Geometry: final body of the model. Coordinates: model frame, mm. A direction names the side the tool comes from. Round coordinates to 2 decimals unless told otherwise and drop trailing zeros. Loops run counter-clockwise (first coordinate to the right, second up) from the corner with the lowest first, then second, coordinate; pieces in that order, holes last. Notation, with made-up numbers: M -21.5,73.5 L 23.5,73.5 A24 cw 23.5,91.5 Z; hole C 83.5,-22.75 d3. An arc over 180 degrees is marked long. Answer as a JSON object with one key per item and string values.
from build123d import *

# Parameters (mm, degrees)
F1_DEPTH = 3
F2_R     = 2.5
F3_DEPTH = 23


with BuildPart() as f1:
    # F0 (on Top) → F1 (new body)
    with BuildSketch(Plane.XY):
        with BuildLine():
            Line((8.3654914829, 7.7478343503), (8.3654914829, 25.7808157751))
            ThreePointArc((8.3654914829, 25.7808157751), (0.4767203504, 33.9966565171), (-7.631576467, 25.9973895632))
            Line((-7.631576467, 25.9973895632), (-8.6528857034, 7.4260866897))
            ThreePointArc((-8.6528857034, 7.4260866897), (-9.3855131516, 5.0826540918), (-11.1453419747, 3.3705145438))
            Line((-11.1453419747, 3.3705145438), (-26.7623619946, -5.6459761686))
            ThreePointArc((-26.7623619946, -5.6459761686), (-29.9331032244, -16.585772745), (-18.951386422, -19.6081302933))
            Line((-18.951386422, -19.6081302933), (-2.3575117339, -11.2069586004))
            ThreePointArc((-2.3575117339, -11.2069586004), (0.038274152, -10.6697162831), (2.400944907, -11.3377029763))
            Line((2.400944907, -11.3377029763), (18.0179649268, -20.3541936886))
            ThreePointArc((18.0179649268, -20.3541936886), (29.0774772891, -17.6302378543), (26.2040573041, -6.6086133521))
            Line((26.2040573041, -6.6086133521), (10.6314918524, 3.5615178285))
            ThreePointArc((10.6314918524, 3.5615178285), (8.9683334147, 5.3677081091), (8.3654914829, 7.7478343503))
        make_face()
        with BuildLine():
            ThreePointArc((-20.451386422, -12.679927063), (-25.3707248656, -13.3098488797), (-20.7688276181, -11.4607318089))
            ThreePointArc((-20.7688276181, -11.4607318089), (-20.5320479783, -12.0500052463), (-20.451386422, -12.679927063))
        make_face(mode=Mode.SUBTRACT)
        with BuildLine():
            ThreePointArc((24.7040573041, -13.5368165824), (21.5399163779, -15.9469860432), (20.0569238399, -12.25626284))
            ThreePointArc((20.0569238399, -12.25626284), (22.8681982302, -11.1266471215), (24.7040573041, -13.5368165824))
        make_face(mode=Mode.SUBTRACT)
        with BuildLine():
            ThreePointArc((-7.9164689421, -4.2812988086), (-7.6979940139, 4.6627125327), (0.127531223, 8.9990963873))
            ThreePointArc((0.127531223, 8.9990963873), (6.4088915191, 6.3187110629), (9, 0))
            ThreePointArc((9, 0), (8.6421794957, -2.5125153857), (7.5971703192, -4.8252464332))
            ThreePointArc((7.5971703192, -4.8252464332), (-0.315369081, -8.9944728774), (-7.9164689421, -4.2812988086))
        make_face(mode=Mode.SUBTRACT)
        with BuildLine():
            ThreePointArc((2.868423533, 25.9973895632), (2.1236210505, 24.217141919), (0.3329981933, 23.4976405667))
            ThreePointArc((0.3329981933, 23.4976405667), (-1.3867739845, 27.7776372074), (2.868423533, 25.9973895632))
        make_face(mode=Mode.SUBTRACT)
        with BuildLine():
            Line((7.5971703192, -4.8252464332), (2.0066709741, -1.4910639161))
            ThreePointArc((2.0066709741, -1.4910639161), (-0.2232494881, -2.4900119811), (-2.239906233, -1.1103243073))
            Line((-2.239906233, -1.1103243073), (-7.9164689421, -4.2812988086))
            ThreePointArc((-7.9164689421, -4.2812988086), (-0.315369081, -8.9944728774), (7.5971703192, -4.8252464332))
        make_face()
        with BuildLine():
            ThreePointArc((-2.239906233, -1.1103243073), (-2.1149683962, 1.333007383), (0.0354253397, 2.4997489965))
            Line((0.0354253397, 2.4997489965), (0.127531223, 8.9990963873))
            ThreePointArc((0.127531223, 8.9990963873), (-7.6979940139, 4.6627125327), (-7.9164689421, -4.2812988086))
            Line((-7.9164689421, -4.2812988086), (-2.239906233, -1.1103243073))
        make_face()
        with BuildLine():
            ThreePointArc((0.0354253397, 2.4997489965), (1.7802476442, 1.7551975175), (2.5, 0))
            ThreePointArc((2.5, 0), (2.3734655501, -0.7852778377), (2.0066709741, -1.4910639161))
            Line((2.0066709741, -1.4910639161), (7.5971703192, -4.8252464332))
            ThreePointArc((7.5971703192, -4.8252464332), (8.6421794957, -2.5125153857), (9, 0))
            ThreePointArc((9, 0), (6.4088915191, 6.3187110629), (0.127531223, 8.9990963873))
            Line((0.127531223, 8.9990963873), (0.0354253397, 2.4997489965))
        make_face()
        with BuildLine():
            ThreePointArc((2.868423533, 25.9973895632), (-1.3867739845, 27.7776372074), (0.3329981933, 23.4976405667))
            ThreePointArc((0.3329981933, 23.4976405667), (2.1236210505, 24.217141919), (2.868423533, 25.9973895632))
        make_face()
        with BuildLine():
            ThreePointArc((24.7040573041, -13.5368165824), (22.8681982302, -11.1266471215), (20.0569238399, -12.25626284))
            ThreePointArc((20.0569238399, -12.25626284), (21.5399163779, -15.9469860432), (24.7040573041, -13.5368165824))
        make_face()
        with BuildLine():
            ThreePointArc((2.0066709741, -1.4910639161), (2.3734655501, -0.7852778377), (2.5, 0))
            ThreePointArc((2.5, 0), (1.7802476442, 1.7551975175), (0.0354253397, 2.4997489965))
            ThreePointArc((0.0354253397, 2.4997489965), (-2.1149683962, 1.333007383), (-2.239906233, -1.1103243073))
            ThreePointArc((-2.239906233, -1.1103243073), (-0.2232494881, -2.4900119811), (2.0066709741, -1.4910639161))
        make_face()
        with BuildLine():
            ThreePointArc((-20.451386422, -12.679927063), (-20.5320479783, -12.0500052463), (-20.7688276181, -11.4607318089))
            ThreePointArc((-20.7688276181, -11.4607318089), (-25.3707248656, -13.3098488797), (-20.451386422, -12.679927063))
        make_face()
    extrude(amount=F1_DEPTH)

    # F2 (on face) → F3 (join)
    with BuildSketch(Plane.XY.offset(3)):
        with Locations((-22.951386422, -12.679927063)):
            Circle(F2_R)
        with Locations((0.368423533, 25.9973895632)):
            Circle(F2_R)
        with Locations((22.2040573041, -13.5368165824)):
            Circle(F2_R)
        Circle(F2_R)
    extrude(amount=F3_DEPTH)


solid = f1.part
1) Section query C-C (z = 9.25). Return the cut outline in (x, y), and give its area (3 significant figures).
Results:
{"outline": "C -22.95,-12.68 d5; C 0,0 d5; C 0.37,26 d5; C 22.2,-13.54 d5", "area": "78.5 mm2"}
2) Pull-direction query (X, two-part tool) for faces 4 (the cylindrical face through (0.043, 28.476, 14.339)), 5 (the cylindrical face through (0, -10.67, 1.48)), 6 (the flat face through (-1, 7, 3)), 7 (the flat face through (-1, 0, 0)); classes: +X half, -X half, draft (parallel to the pull), parting line (faces both ways), or undercut.
Results:
{"face 4": "parting line", "face 5": "undercut", "face 6": "undercut", "face 7": "draft"}
3) Reachability of faces 1 (the flat face through (-10.771, -15.466, 1.479)), 2 (the cylindrical face through (-20.642, -13.637, 14.339)), 3 (the flat face through (0, 26, 26)) from +Z, -Z, +X, -X, +Y, -Y: full face, straight path, thin tool, end or side. Return the list, or none.
Results:
{"face 1": "+Z, -Z, -Y", "face 2": "+Z", "face 3": "+Z, +X, -X, +Y, -Y"}
4) Section query D-D (y = 0). Return the cut outline in (x, z).
Results:
{"outline": "M -16.98,0 L 16.08,0 L 16.08,3 L 2.5,3 L 2.5,26 L -2.5,26 L -2.5,3 L -16.98,3 Z"}
5) Pin query (flat end, axial travel): P1, Ø6, axis at y = 26.5, z = 21, coming from the +X side; P2, Ø8, axis at x = -3.5, z = 5, coming from the +Y side; P3, Ø2.5, axis at y = 21, z = 1, coming from the +X side. Return the tip coordinate at first contact, or that it passes through.
Results:
{"P1": "x = 2.87", "P2": "y = 33.99", "P3": "x = 8.37"}
6) Section query A-A (y = -17). Return the cut outline in (x, z), and give its area (3 significant figures).
Results:
{"outline": "M -29.68,0 L -13.8,0 L -13.8,3 L -29.68,3 Z; M 12.21,0 L 29.42,0 L 29.42,3 L 12.21,3 Z", "area": "99.3 mm2"}
7) Ray query, line 1 (Z direction, x = -6, y = 13); line 2 (Y direction, x = 1, z = 9.5); line 3 (Y direction, x = -21, z = 15.75). Return the intervals inside material, ascending.
Results:
{"line 1": "0 to 3", "line 2": "-2.29 to 2.29, 23.58 to 28.42", "line 3": "-14.24 to -11.12"}
8) Section query B-B (x = -23.5). Return the cut outline in (y, z), and give its area (3 significant figures).
Results:
{"outline": "M -20.66,0 L -3.76,0 L -3.76,3 L -10.24,3 L -10.24,26 L -15.12,26 L -15.12,3 L -20.66,3 Z", "area": "163 mm2"}
